Check sheet for the modelled part. Datum: model origin and axes. Units: mm. A direction names the side the tool comes from. Coordinates: 2 decimals unless noted, no trailing zeros. Loops run counter-clockwise (first coordinate to the right, second up) from the corner with the lowest first, then second, coordinate; pieces in that order, holes last.
from build123d import *

# Parameters (mm, degrees)
SKETCH004_AS_DRAWN_W                 = 6
SKETCH004_AS_DRAWN_H                 = 52
EXTRUDE003_DEPTH                     = 15
EXTRUDE003_ONTO_SKETCH004_ROLL_ANGLE = 90
EXTRUDE002_DEPTH                     = 167
EXTRUDE001_DEPTH                     = 3
SKETCH_R                             = 4.6875
EXTRUDE_DEPTH                        = 3


with BuildPart() as extrude003:
    # Sketch004 as drawn → Extrude003 (new)
    with BuildSketch(Plane.XY):
        with Locations((-74.75, 29)):
            Rectangle(SKETCH004_AS_DRAWN_W, SKETCH004_AS_DRAWN_H)
        with Locations((-63.25, 29)):
            Rectangle(SKETCH004_AS_DRAWN_W, SKETCH004_AS_DRAWN_H)
        with Locations((-51.75, 29)):
            Rectangle(SKETCH004_AS_DRAWN_W, SKETCH004_AS_DRAWN_H)
        with Locations((-40.25, 29)):
            Rectangle(SKETCH004_AS_DRAWN_W, SKETCH004_AS_DRAWN_H)
        with Locations((-28.75, 29)):
            Rectangle(SKETCH004_AS_DRAWN_W, SKETCH004_AS_DRAWN_H)
        with Locations((-17.25, 29)):
            Rectangle(SKETCH004_AS_DRAWN_W, SKETCH004_AS_DRAWN_H)
        with Locations((-5.75, 29)):
            Rectangle(SKETCH004_AS_DRAWN_W, SKETCH004_AS_DRAWN_H)
        with Locations((5.75, 29)):
            Rectangle(SKETCH004_AS_DRAWN_W, SKETCH004_AS_DRAWN_H)
        with Locations((17.25, 29)):
            Rectangle(SKETCH004_AS_DRAWN_W, SKETCH004_AS_DRAWN_H)
        with Locations((28.75, 29)):
            Rectangle(SKETCH004_AS_DRAWN_W, SKETCH004_AS_DRAWN_H)
        with Locations((40.25, 29)):
            Rectangle(SKETCH004_AS_DRAWN_W, SKETCH004_AS_DRAWN_H)
        with Locations((51.75, 29)):
            Rectangle(SKETCH004_AS_DRAWN_W, SKETCH004_AS_DRAWN_H)
        with Locations((63.25, 29)):
            Rectangle(SKETCH004_AS_DRAWN_W, SKETCH004_AS_DRAWN_H)
        with Locations((74.75, 29)):
            Rectangle(SKETCH004_AS_DRAWN_W, SKETCH004_AS_DRAWN_H)
    extrude(amount=-EXTRUDE003_DEPTH)


with BuildPart() as extrude003_1:
    # Extrude003 onto Sketch004 roll: moved
    add(extrude003.part.rotate(Axis((0, 0, 0), (1, 0, 0)), EXTRUDE003_ONTO_SKETCH004_ROLL_ANGLE))


with BuildPart() as extrude003_2:
    # Extrude003 onto Sketch004 placement: moved
    add(extrude003_1.part.moved(Location((0, -10, 0))))


with BuildPart() as cut001:
    # Sketch003 → Extrude002 (new body)
    with BuildSketch(Plane(origin=(-83.5, 0, 0), x_dir=(0, -1, 0), z_dir=(-1, 0, 0))):
        Polygon((0, 55), (-5, 55), (-3, 49), (-3, 3), (10, 3), align=None)
    extrude(amount=-EXTRUDE002_DEPTH)

    # Cut001: cut Extrude003
    add(extrude003_2.part, mode=Mode.SUBTRACT)


with BuildPart() as extrude001:
    # Sketch001 → Extrude001 (new body)
    with BuildSketch(Plane.XY.offset(3)):
        with BuildLine():
            ThreePointArc((-54.05, 10), (-50.8, 6.75), (-47.55, 10))
            Line((-47.55, 10), (-47.55, 20))
            ThreePointArc((-47.55, 20), (-50.8, 23.25), (-54.05, 20))
            Line((-54.05, 10), (-54.05, 20))
        make_face()
        with BuildLine():
            ThreePointArc((47.55, 10), (50.8, 6.75), (54.05, 10))
            Line((54.05, 10), (54.05, 20))
            ThreePointArc((54.05, 20), (50.8, 23.25), (47.55, 20))
            Line((47.55, 10), (47.55, 20))
        make_face()
    extrude(amount=-EXTRUDE001_DEPTH)


with BuildPart() as fusion:
    # Sketch → Extrude (new body)
    with BuildSketch(Plane.XY):
        with BuildLine():
            Line((-83.5, 20), (-83.5, -10))
            Line((-83.5, -10), (83.5, -10))
            Line((83.5, -10), (83.5, 20))
            ThreePointArc((83.5, 20), (80.566817, 27.075323), (73.487973, 30))
            Line((-73.500027, 30), (73.487973, 30))
            ThreePointArc((-73.500027, 30), (-80.571077, 27.071058), (-83.5, 20))
        make_face()
        with Locations((50.8, 10)):
            Circle(SKETCH_R, mode=Mode.SUBTRACT)
        with Locations((-50.8, 10)):
            Circle(SKETCH_R, mode=Mode.SUBTRACT)
    extrude(amount=EXTRUDE_DEPTH)

    # Cut: cut Extrude001
    add(extrude001.part, mode=Mode.SUBTRACT)

    # Fusion: union Cut001
    add(cut001.part)


solid = fusion.part
(1) Section check B-B, the plane y = 18.5. Enter the section's corners in (x, z), plus the area to 3 significant figures.
(2) Section check C-C, the plane y = 10. Enter the section's corners in (x, z).
(3) Scan lines: line 1 along X through (y, z) = (10, 2.05); line 2 along Y through (x, z) = (50.8, 2.2); line 3 along Z through (x, y) = (12.5, 11.5). Record each from-to range of solid material in increasing order.
(4) Section check A-A, the plane x = -50.8. Enter the section's corners in (y, z), plus the area to 3 significant figures.
(5) Gauge pin test, flat ends, axial feed: P1, Ø8, axis at x = -24.5, z = 10.5, coming from the +Y side; P2, Ø5, axis at x = -27.5, z = 44.5, coming from the -Y side; P3, Ø1, axis at x = 11, z = 44.5, coming from the -Y side. Record the tip position at first contact, or that the pin passes through.
(6) Draft check along X on faces 6 (the face through (37.25, -1, 23)), 7 (the face through (-23, 4, 52)). Enter one of: pulls with the +X half, pulls with the -X half, needs draft (parallel to the pull), parting line crosses it, or undercut.
(7) Section check D-D, the plane x = 5.5. Enter the section's corners in (y, z).
(8) Set-up check for faces 1 (the face through (-50.73, 23.25, 1.52)), 2 (the face through (23, 4, 52)), 3 (the face through (-25.75, -1, 23)), 4 (the face through (46, -5, 29)), 5 (the face through (81, 2, 55)): record each of +Z, -Z, +X, -X, +Y, -Y from which the full face is reachable in a straight line by a thin tool's end or side.
Determined:
1. outline: (-83.5, 0) - (-54.05, 0) - (-54.05, 3) - (-83.5, 3) - close; (-47.55, 0) - (47.55, 0) - (47.55, 3) - (-47.55, 3) - close; (54.05, 0) - (83.5, 0) - (83.5, 3) - (54.05, 3) - close
1. area: 462 mm2
2. outline: (-83.5, 0) - (-55.49, 0) - (-55.49, 3) - (-83.5, 3) - close; (-46.11, 0) - (46.11, 0) - (46.11, 3) - (-46.11, 3) - close; (55.49, 0) - (83.5, 0) - (83.5, 3) - (55.49, 3) - close
3. line 1: x = -83.5 to -55.49, -46.11 to 46.11, 55.49 to 83.5
3. line 2: y = -10 to 5.31, 23.25 to 30
3. line 3: z = 0 to 3
4. outline: (-10, 0) - (5.31, 0) - (5.31, 3) - (-10, 3) - close; (23.25, 0) - (30, 0) - (30, 3) - (23.25, 3) - close
4. area: 66.2 mm2
5. P1: stops at y = 3
5. P2: stops at y = -2.36
5. P3: stops at y = -2.12
6. face 6: undercut
6. face 7: needs draft
7. outline: (-10, 0) - (30, 0) - (30, 3) - (-10, 3) - close
8. face 1: +Z, -Z
8. face 2: +X, -X, +Y
8. face 3: +Z, +Y, -Y
8. face 4: +Z, +X, -X, -Y
8. face 5: +Z, +X, -X, +Y, -Y
